from build123d import *

# Parameters (mm, degrees)
SKETCH1_W           = 25.4
SKETCH1_H           = 6.35
BOSS_EXTRUDE1_DEPTH = 100
SKETCH2_R           = 2.1
CUT_EXTRUDE1_DEPTH  = 110.906322202
SKETCH2_3_R         = 5
CUT_EXTRUDE2_DEPTH  = 4
SKETCH2_4_R         = 5
CUT_EXTRUDE3_DEPTH  = 4
SKETCH5_W           = 25.4
SKETCH5_H           = 5
SKETCH5_H_2         = 12
CUT_EXTRUDE4_DEPTH  = 110.906322202
SKETCH6_W           = 25.4
SKETCH6_H           = 3.7
CUT_EXTRUDE5_DEPTH  = 106.377415322


with BuildPart() as part:
    # Sketch1 → Boss-Extrude1 (new body)
    with BuildSketch(Plane(origin=(0, 0, 0), x_dir=(1, 0, 0), z_dir=(0, 1, 0))):
        with Locations((32.456141995, 0.058688594)):
            Rectangle(SKETCH1_W, SKETCH1_H)
    extrude(amount=BOSS_EXTRUDE1_DEPTH)

    # Sketch2 → Cut-Extrude1 (cut, through all)
    with BuildSketch(Plane.XY.offset(3.116311406)):
        with Locations((32.456141995, 81.7)):
            Circle(SKETCH2_R)
        with Locations((32.456141995, 23.71)):
            Circle(SKETCH2_R)
    extrude(amount=-CUT_EXTRUDE1_DEPTH, mode=Mode.SUBTRACT)

    # Sketch2<3> → Cut-Extrude2 (cut)
    with BuildSketch(Plane.XY.offset(3.116311406)):
        with Locations((32.456141995, 81.7)):
            Circle(SKETCH2_3_R)
    extrude(amount=-CUT_EXTRUDE2_DEPTH, mode=Mode.SUBTRACT)

    # Sketch2<4> → Cut-Extrude3 (cut)
    with BuildSketch(Plane.XY.offset(3.116311406)):
        with Locations((32.456141995, 23.71)):
            Circle(SKETCH2_4_R)
    extrude(amount=-CUT_EXTRUDE3_DEPTH, mode=Mode.SUBTRACT)

    # Sketch5 → Cut-Extrude4 (cut, through all)
    with BuildSketch(Plane.XY.offset(3.116311406)):
        with Locations((32.456141995, 97.5)):
            Rectangle(SKETCH5_W, SKETCH5_H)
        with Locations((32.456141995, 6)):
            Rectangle(SKETCH5_W, SKETCH5_H_2)
    extrude(amount=-CUT_EXTRUDE4_DEPTH, mode=Mode.SUBTRACT)

    # Sketch6 → Cut-Extrude5 (cut, through all)
    with BuildSketch(Plane.XY.offset(3.116311406)):
        with Locations((32.456141995, 13.85)):
            Rectangle(SKETCH6_W, SKETCH6_H)
    extrude(amount=-CUT_EXTRUDE5_DEPTH, mode=Mode.SUBTRACT)


solid = part.part
Can you work these out from the model? Positions are in its coordinate system, mm. A direction names the side the tool comes from. Give positions to 0.01 mm unless a question says otherwise; leave off trailing zeros. Order: outer loops, then holes, each group sorted by start corner. A loop starts at its lowest first (then second) coordinate and runs counter-clockwise, first axis right, second up. Notation, with made-up numbers: M -28,74 L -16,74 A17 ccw -16,99 Z; hole C -19,-5.75 d7. An arc over 180 degrees is marked long. Use a Markdown table: item, result. Add a question column.
Item 1: Suppose I cut it at A-A (y = 81.7). List the corners of the cut face in (x, z) for me.
Item 2: Suppose I cut it at B-B (z = 1.5). List the corners of the cut face in (x, y) for me.
Item 3: Will this pin go through, and if not, where does the flat tip stop? pin 1 (5 mm diameter, centred on x = 32.46, y = 23.71, fed in from +Z).
Item 4: We'd pull the mould along X, two halves only. Please class faces 1 (the cylindrical face through (30.91, 25.13, -2.04)), 2 (the flat face through (32, 95, 0)), 3 (the flat face through (19.756, 55, 0)): +X half, -X half, draft (parallel to the pull), parting line (faces both ways), or undercut.
Item 5: Suppose I cut it at C-C (x = 31.5). List the corners of the cut face in (y, z) for me, then the cut area to 3 significant figures.
Item 6: For faces 4 (the flat face through (45.156, 55, 0)), 5 (the flat face through (35, 24, -0.884)), which set-ups out of +Z, -Z, +X, -X, +Y, -Y let a thin tool reach every point of the face, with its end or its side?
Item 7: If I drill on L1, parallel to Y at x = 37, z = 1.5; L2, parallel to Y at x = 30.25, z = 1.5; L3, parallel to X at y = 85.5, z = 1, over which ranges is the centre line in solid material (lowest first)? Write a range as [from, to].
Answer sheet:
| question | item | result |
|---|---|---|
| 1 | outline | M 19.76,-3.23 L 30.36,-3.23 L 30.36,-0.88 L 27.46,-0.88 L 27.46,3.12 L 19.76,3.12 Z; M 34.56,-3.23 L 45.16,-3.23 L 45.16,3.12 L 37.46,3.12 L 37.46,-0.88 L 34.56,-0.88 Z |
| 2 | outline | M 19.76,15.7 L 45.16,15.7 L 45.16,95 L 19.76,95 Z; hole C 32.46,23.71 d10; hole C 32.46,81.7 d10 |
| 3 | pin 1 | stops at z = -0.88 |
| 4 | face 1 | undercut |
| 4 | face 2 | draft |
| 4 | face 3 | -X half |
| 5 | outline | M 15.7,-3.23 L 21.84,-3.23 L 21.84,-0.88 L 18.8,-0.88 L 18.8,3.12 L 15.7,3.12 Z; M 25.58,-3.23 L 79.83,-3.23 L 79.83,-0.88 L 76.79,-0.88 L 76.79,3.12 L 28.62,3.12 L 28.62,-0.88 L 25.58,-0.88 Z; M 83.57,-3.23 L 95,-3.23 L 95,3.12 L 86.61,3.12 L 86.61,-0.88 L 83.57,-0.88 Z |
| 5 | area | 407 mm² |
| 6 | face 4 | +Z, -Z, +X, +Y, -Y |
| 6 | face 5 | +Z |
| 7 | L1 | y = [15.7, 21.62], [25.8, 79.61], [83.79, 95] |
| 7 | L2 | y = [15.7, 19.22], [28.2, 77.21], [86.19, 95] |
| 7 | L3 | x = [19.76, 29.21], [35.71, 45.16] |
